Autodesk Inventor part; units mm, degrees
ref_plane "YZ Plane" through (0, 0, 0) normal (1, 0, 0) x (0, 1, 0)
ref_plane "XZ Plane" through (0, 0, 0) normal (0, 1, 0) x (-1, 0, 0)
ref_plane "XY Plane" through (0, 0, 0) normal (0, 0, 1) x (1, 0, 0)
sketch "スケッチ1" plane through (0, 0, 0) normal (0, 0, 1) x (1, 0, 0)
  line L0 (0, 0) -> (20, 0)
  line L1 (20, 0) -> (20, 30)
  line L2 (20, 30) -> (0, 30)
  line L3 (0, 30) -> (0, 0)
  dimension "d0" = 20
  dimension "d1" = 30
extrude "押し出し1" add sketch "スケッチ1" along normal blind 10
sketch "スケッチ2" plane through (0, 0, 10) normal (0, 0, 1) x (1, 0, 0)
  line L0 (0, 0) -> (20, 0)
  line L1 (10, 0) -> (10, 6.3032)
  point P0 (3, 5)
  point P1 (17, 5)
  dimension "d4" = 5
  dimension "d5" = 7
hole "穴1" at (3, 5, 10) at (17, 5, 10) direction (0, 0, -1) diameter 3 end through all
sketch "スケッチ3" plane through (0, 0, 10) normal (0, 0, 1) x (1, 0, 0)
  line L0 (20, 30) -> (0, 30)
  line L1 (0, 30) -> (20, 10)
  line L2 (20, 0) -> (20, 30)
  point P0 (0, 0)
  dimension "d13" = 10
properties part number "指上"
Design review of the part built by this model. Coordinates are the model's own, in mm. Coordinates: 2 decimals unless noted, no trailing zeros. Order: outer loops, then holes, each group sorted by start corner. A loop starts at its lowest first (then second) coordinate and runs counter-clockwise, first axis right, second up. Notation, with made-up numbers: M 7.25,-33 L 38.25,-33 A18 cw 38.25,-23 Z; hole C 31.5,53 d1. An arc over 180 degrees is marked long. Answer as a JSON object with one key per item and string values. Group by question number.
1) Add section C-C, the plane z = 1. Write out the cut boundary in (x, y), then the cut area to 3 significant figures.
2) Wall thickness on L1, parallel to X at y = 5, z = 4; L2, parallel to Y at x = 3, z = 5; L3, parallel to X at y = 4.5, z = 4.5: over which ranges is each line inside the solid? List them lowest first.
3) Add section B-B, the plane y = 5. Write out the cut boundary in (x, z), then the cut area to 3 significant figures.
4) Mouldability with a two-part tool opening along Y and no side actions: class faces 1 (the cylindrical face through (15.99, 6.11, 4.93)), 2 (the flat face through (20, 15, 5)), 3 (the flat face through (10, 30, 5)) as pulls with the +Y half, pulls with the -Y half, needs draft (parallel to the pull), parting line crosses it, or undercut.
5) For pin 1 (2.5 mm diameter, centred on x = 17, y = 5, fed in from -Z), flat-tipped, find the tip position at first contact; note if it passes through.
6) Add section A-A, the plane x = 3. Write out the cut boundary in (y, z).
Computed values:
{
 "1": {"outline": "M 0,0 L 20,0 L 20,30 L 0,30 Z; hole C 3,5 d3; hole C 17,5 d3", "area": "586 mm^2"},
 "2": {"L1": "x = 0 to 1.5, 4.5 to 15.5, 18.5 to 20", "L2": "y = 0 to 3.5, 6.5 to 30", "L3": "x = 0 to 1.59, 4.41 to 15.59, 18.41 to 20"},
 "3": {"outline": "M 0,0 L 1.5,0 L 1.5,10 L 0,10 Z; M 4.5,0 L 15.5,0 L 15.5,10 L 4.5,10 Z; M 18.5,0 L 20,0 L 20,10 L 18.5,10 Z", "area": "140 mm^2"},
 "4": {"face 1": "undercut", "face 2": "needs draft", "face 3": "pulls with the +Y half"},
 "5": {"pin 1": "passes through"},
 "6": {"outline": "M 0,0 L 3.5,0 L 3.5,10 L 0,10 Z; M 6.5,0 L 30,0 L 30,10 L 6.5,10 Z"}
}
